Design review of the part built by this model. Coordinates are the model's own, in mm. Face numbers are marked on the shaded views. A direction names the side the tool comes from. Round coordinates to 2 decimals unless told otherwise and drop trailing zeros. Write each loop counter-clockwise with the first axis right and the second up, starting at its lowest first coordinate (ties: lowest second). Pieces come first, ordered by that corner, then holes. Notation, with made-up numbers: M 17,21.5 L 28,21.5 A15 ccw 28,41.5 Z; hole C 37,8.25 d10. An arc over 180 degrees is marked long. One line per question, with ' | ' between items. Start each with the question number.
Item 1: Add section D-D, the plane y = -5. State the section outline as (x, z) points, and give its area (3 significant figures).
Item 2: Add section A-A, the plane y = 33. State the section outline as (x, z) points, and give its area (3 significant figures).
Item 3: Draft analysis for pull direction X (two halves, no side actions). For the marked faces 1, 2 and 3, state which applies: released by +X, released by -X, zero draft, split by the parting line, or undercut.
Item 4: For L1, parallel to Y at x = -65.5, z = 1.45; L2, parallel to X at y = 32.5, z = 6.5; L3, parallel to Z at x = -17, y = 36.5, list the stretches that pass through material, from the lowest coordinate up.
Item 5: Add section B-B, the plane x = -65.5. State the section outline as (y, z) points.
Item 6: Machinability: for the marked faces 4, 5, 6 and 7, which of the approach directions +Z, -Z, +X, -X, +Y, -Y give a long, thin tool a straight path to every point of the face, cutting with its end or side? Answer none if there is none.
Item 7: Insertion check: pin 1 Ø6 at (y, z) = (-28, 10.5) entering from -X; pin 2 Ø8 at (x, z) = (14, 14) entering from +Y; pin 3 Ø4 at (y, z) = (36.5, 12) entering from +X; pin 4 Ø1.8 at (x, y) = (65.5, -33) entering from +Z. Each pin has a flat end and moves straight along its axis. Give the tip position at first contact, or say it passes through.
Item 8: Add section C-C, the plane z = 10.75. State the section outline as (x, y) points, and give its area (3 significant figures).
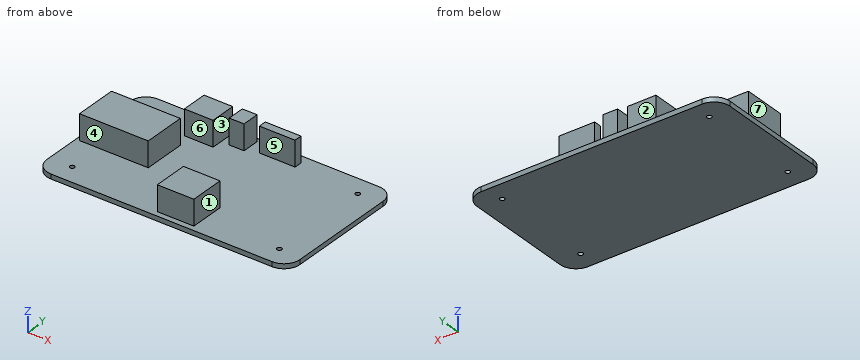
```python
from build123d import *

# Parameters (mm, degrees)
SKETCH1_W           = 160
SKETCH1_H           = 90
BOSS_EXTRUDE1_DEPTH = 3
FILLET1_R           = 10
SKETCH2_R           = 1.5
CUT_EXTRUDE1_DEPTH  = 4
SKETCH3_W           = 43.515917568
SKETCH3_H           = 26.99088558
SKETCH3_W_2         = 23.135044783
SKETCH3_H_2         = 22.033375984
SKETCH3_W_3         = 18.177535187
SKETCH3_H_3         = 16.525031987
SKETCH3_W_4         = 9.364184793
SKETCH3_H_4         = 11.016687992
SKETCH3_W_5         = 22.584210384
SKETCH3_H_5         = 4.957509597
BOSS_EXTRUDE2_DEPTH = 16


with BuildPart() as part:
    # Sketch1 → Boss-Extrude1 (new body)
    with BuildSketch(Plane.XY):
        Rectangle(SKETCH1_W, SKETCH1_H)
    extrude(amount=BOSS_EXTRUDE1_DEPTH)

    # Fillet1
    fillet1_edges = [part.edges().sort_by_distance(p)[0] for p in [
        (80, -45, 1.5),
        (-80, -45, 1.5),
        (-80, 45, 1.5),
        (80, 45, 1.5),
    ]]
    fillet(fillet1_edges, radius=FILLET1_R)

    # Sketch2 → Cut-Extrude1 (cut, through all)
    with BuildSketch(Plane.XY.offset(3)):
        with Locations((-65.5, 33)):
            Circle(SKETCH2_R)
        with Locations((65.5, 33)):
            Circle(SKETCH2_R)
        with Locations((65.5, -33)):
            Circle(SKETCH2_R)
        with Locations((-65.5, -33)):
            Circle(SKETCH2_R)
    extrude(amount=-CUT_EXTRUDE1_DEPTH, mode=Mode.SUBTRACT)

    # Sketch3 → Boss-Extrude2 (add)
    with BuildSketch(Plane.XY.offset(3)):
        with Locations((-55.967549569, 2.815480553)):
            Rectangle(SKETCH3_W, SKETCH3_H)
        with Locations((6.276737585, -30.510000623)):
            Rectangle(SKETCH3_W_2, SKETCH3_H_2)
        with Locations((-28.976663989, 33.111372531)):
            Rectangle(SKETCH3_W_3, SKETCH3_H_3)
        with Locations((-9.972877203, 36.967213328)):
            Rectangle(SKETCH3_W_4, SKETCH3_H_4)
        with Locations((13.43758478, 36.967213328)):
            Rectangle(SKETCH3_W_5, SKETCH3_H_5)
    extrude(amount=BOSS_EXTRUDE2_DEPTH)


solid = part.part
```
Computed values:
1) outline: M -80,0 L 80,0 L 80,3 L -34.21,3 L -34.21,19 L -77.73,19 L -77.73,3 L -80,3 Z | area: 1,180 mm^2
2) outline: M -80,0 L -67,0 L -67,3 L -80,3 Z; M -64,0 L 64,0 L 64,3 L -5.29,3 L -5.29,19 L -14.65,19 L -14.65,3 L -19.89,3 L -19.89,19 L -38.07,19 L -38.07,3 L -64,3 Z; M 67,0 L 80,0 L 80,3 L 67,3 Z | area: 903 mm^2
3) face 1: released by +X | face 2: zero draft | face 3: undercut
4) L1: y = -45 to -34.5, -31.5 to 31.5, 34.5 to 45 | L2: x = -38.07 to -19.89, -14.65 to -5.29 | L3: z = 0 to 3
5) outline: M -45,0 L -34.5,0 L -34.5,3 L -45,3 Z; M -31.5,0 L 31.5,0 L 31.5,3 L 16.31,3 L 16.31,19 L -10.68,19 L -10.68,3 L -31.5,3 Z; M 34.5,0 L 45,0 L 45,3 L 34.5,3 Z
6) face 4: +Z, +X, -X, -Y | face 5: +Z, +X | face 6: +Z, +X, -X | face 7: +Z, -X, +Y, -Y
7) pin 1: stops at x = -5.29 | pin 2: stops at y = 39.45 | pin 3: stops at x = 24.73 | pin 4: passes through
8) outline: M -77.73,-10.68 L -34.21,-10.68 L -34.21,16.31 L -77.73,16.31 Z; M -38.07,24.85 L -19.89,24.85 L -19.89,41.37 L -38.07,41.37 Z; M -14.65,31.46 L -5.29,31.46 L -5.29,42.48 L -14.65,42.48 Z; M -5.29,-41.53 L 17.84,-41.53 L 17.84,-19.49 L -5.29,-19.49 Z; M 2.15,34.49 L 24.73,34.49 L 24.73,39.45 L 2.15,39.45 Z | area: 2,200 mm^2
